from build123d import *

# Parameters (mm, degrees)
ESQUISSE1_R             = 1.5
BOSS_EXTRU_1_DEPTH      = 5
CONG_1_R                = 0.2
ESQUISSE2_R             = 1.4
ENL_V_MAT_EXTRU_1_DEPTH = 0.02
ESQUISSE3_R             = 0.6
BOSS_EXTRU_2_DEPTH      = 10


with BuildPart() as part:
    # Esquisse1 → Boss.-Extru.1 (new body)
    with BuildSketch(Plane.XY):
        Circle(ESQUISSE1_R)
    extrude(amount=BOSS_EXTRU_1_DEPTH)

    # Congé1
    cong_1_edges = [part.edges().sort_by_distance(p)[0] for p in [
        (-1.5, 0, 0),
    ]]
    fillet(cong_1_edges, radius=CONG_1_R)

    # Esquisse2 → Enlèv. mat.-Extru.1 (cut)
    with BuildSketch(Plane.XY.offset(5)):
        Circle(ESQUISSE2_R)
    extrude(amount=-ENL_V_MAT_EXTRU_1_DEPTH, mode=Mode.SUBTRACT)

    # Esquisse3 → Boss.-Extru.2 (add)
    with BuildSketch(Plane.XY.offset(4.98)):
        with Locations((-0.7, 0)):
            Circle(ESQUISSE3_R)
        with Locations((0.7, 0)):
            Circle(ESQUISSE3_R)
    extrude(amount=BOSS_EXTRU_2_DEPTH)


solid = part.part
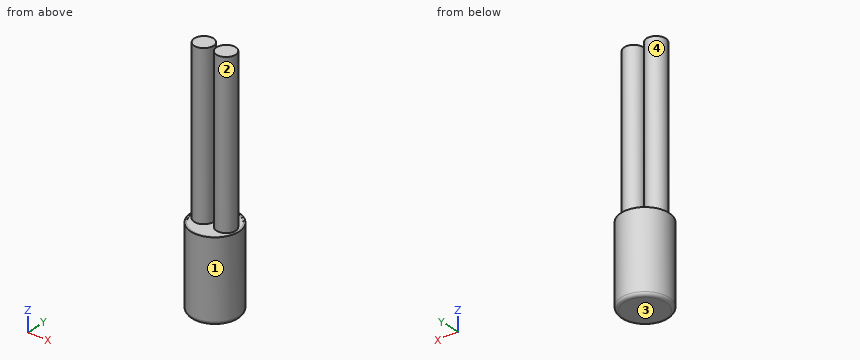
Check sheet for the modelled part. Datum: model origin and axes. Units: mm. Face numbers are marked on the shaded views. Give positions to 0.01 mm unless a question says otherwise; leave off trailing zeros. Write each loop counter-clockwise with the first axis right and the second up, starting at its lowest first coordinate (ties: lowest second). Pieces come first, ordered by that corner, then holes. Notation, with made-up numbers: (-27.75, 32.5) -> (25.25, 32.5) arc R30 ccw to (25.25, 64.5) -> close; hole circle Ø7 at (-20.75, 68.5). An arc over 180 degrees is marked (long way). One line per item, written item: value. Start each with the question number.
Item 1: Draft check along X on the marked faces 1, 2, 3 and 4. Enter one of: +X half, -X half, draft (parallel to the pull), parting line (faces both ways), or undercut.
Item 2: Section check C-C on z = 3. Record the cut outline in (x, y), then the cut area to 3 significant figures.
Item 3: Section check B-B on z = 10.5. Record the cut outline in (x, y), then the cut area to 3 significant figures.
Item 4: Material ranges on probe 1 along Z at (x, y) = (-0.8, 0.95); probe 2 along X at (y, z) = (0.4, 11.5); probe 3 along Y at (x, z) = (-0.9, 6), recorded low to high. Write a range as from..to.
Item 5: Gauge pin test, flat end, axial feed: pin 1 (1.5 mm diameter, centred on y = -1, z = 6, fed in from -X). Record the tip position at first contact, or that the pin passes through.
Results list:
1. face 1: parting line
1. face 2: undercut
1. face 3: draft
1. face 4: undercut
2. outline: circle Ø3 at (0, 0)
2. area: 7.07 mm²
3. outline: circle Ø1.2 at (-0.7, 0); circle Ø1.2 at (0.7, 0)
3. area: 2.26 mm²
4. probe 1: 0..4.98
4. probe 2: -1.15..-0.25, 0.25..1.15
4. probe 3: -0.57..0.57
5. pin 1: x = -1.25
